Could you check a few things on this model? Use its own coordinates, in mm. A direction names the side the tool comes from. Coordinates: 2 decimals unless noted, no trailing zeros. Write each loop counter-clockwise with the first axis right and the second up, starting at its lowest first coordinate (ties: lowest second). Pieces come first, ordered by that corner, then holes.
Autodesk Inventor part; units mm, degrees
ref_plane "YZ Plane" through (0, 0, 0) normal (1, 0, 0) x (0, 1, 0)
ref_plane "XZ Plane" through (0, 0, 0) normal (0, 1, 0) x (-1, 0, 0)
ref_plane "XY Plane" through (0, 0, 0) normal (0, 0, 1) x (1, 0, 0)
sketch "Sketch1" plane through (0, 0, 0) normal (0, 0, 1) x (1, 0, 0)
  arc A0 (-25.4018, -15) -> (25.4018, -15) centre (0, 0) ccw
  line L0 (2.5, -32) -> (2.5, -39)
  line L1 (2.5, -39) -> (-2.5, -39)
  line L2 (-2.5, -39) -> (-2.5, -32)
  line L3 (-2.5, -32) -> (-2.5, -31.9022)
  line L4 (2.5, -32) -> (2.5, -31.9022)
  arc A1 (-28.2666, -15) -> (-2.5, -31.9022) centre (0, 0) ccw
  arc A2 (2.5, -31.9022) -> (28.2666, -15) centre (0, 0) ccw
  line L5 (-28.2666, -15) -> (-25.4018, -15)
  line L6 (25.4018, -15) -> (28.2666, -15)
  dimension "d43" = 5
  dimension "d64" = 7
extrude "Extrusion5" add sketch "Sketch1" along normal blind 5
properties part number "Clip_TestFitV1"
Item 1: I want a section at D-D, the plane x = 10.5. List the corners of the cut face in (y, z) for me, then the cut area to 3 significant figures.
Item 2: If I drill on line 1 along X through (y, z) = (-33.75, 1.1); line 2 along X through (y, z) = (-17.75, 0.6); line 3 along X through (y, z) = (-18.25, 2.45), over which ranges is the centre line in solid material (lowest first)?
Item 3: I want a section at B-B, the plane z = 2.8. List the corners of the cut face in (x, y) for me.
Item 4: Which directions (+Z, -Z, +X, -X, +Y, -Y) give clear straight access to the entire face, cutting with the end or side of a thin tool? Please do faces 4 (the flat face through (-2.5, -36, 2)), 5 (the flat face through (27, -15, 2)).
Item 5: I want a section at C-C, the plane y = -28. List the corners of the cut face in (x, z) for me, then the cut area to 3 significant figures.
Item 6: Will these pins go through, and if not, where does the flat tip stop? pin 1 Ø1 at (x, z) = (4.5, 4.5) entering from -Y; pin 2 Ø2.5 at (y, z) = (-35.5, 2.5) entering from +X; pin 3 Ø2 at (y, z) = (-28, 4.5) entering from +X.
Item 7: I want a section at A-A, the plane y = -21.25. List the corners of the cut face in (x, z) for me.
Item 8: If we mould it in two halves opening along X, with no side actions, what happens to faces 1 (the cylindrical face through (0.428, -29.497, 2.465)), 2 (the flat face through (2.5, -35, 2)), 3 (the flat face through (0, -39, 2))? For each: released by +X, released by -X, zero draft, split by the parting line, or undercut.
Taken from the geometry:
1. outline: (-30.23, 0) - (-27.57, 0) - (-27.57, 5) - (-30.23, 5) - close
1. area: 13.3 mm2
2. line 1: x = -2.5 to 2.5
2. line 2: x = -26.63 to -23.56, 23.56 to 26.63
2. line 3: x = -26.29 to -23.18, 23.18 to 26.29
3. outline: (-28.27, -15) arc R32 ccw to (-2.5, -31.9) - (-2.5, -39) - (2.5, -39) - (2.5, -31.9) arc R32 ccw to (28.27, -15) - (25.4, -15) arc R29.5 cw to (-25.4, -15) - close
4. face 4: +Z, -Z, -X, -Y
4. face 5: +Z, -Z, +X, -X, +Y
5. outline: (-15.49, 0) - (-9.29, 0) - (-9.29, 5) - (-15.49, 5) - close; (9.29, 0) - (15.49, 0) - (15.49, 5) - (9.29, 5) - close
5. area: 62.0 mm2
6. pin 1: stops at y = -31.75
6. pin 2: stops at x = 2.5
6. pin 3: stops at x = 17.18
7. outline: (-23.93, 0) - (-20.46, 0) - (-20.46, 5) - (-23.93, 5) - close; (20.46, 0) - (23.93, 0) - (23.93, 5) - (20.46, 5) - close
8. face 1: undercut
8. face 2: released by +X
8. face 3: zero draft
